from build123d import *

# Parameters (mm, degrees)
BOSS_EXTRUDE1_DEPTH = 7.9
SKETCH2_R           = 3.144549921
BOSS_EXTRUDE3_DEPTH = 0.5
SKETCH3_R           = 2.455888386
BOSS_EXTRUDE4_DEPTH = 7.9
SKETCH4_R           = 2.65462565
BOSS_EXTRUDE5_DEPTH = 0.3
SKETCH5_R           = 2.198604039
CUT_EXTRUDE1_DEPTH  = 7.9
CUT_EXTRUDE2_DEPTH  = 3.3
FILLET1_R           = 0.3
CUT_EXTRUDE5_START  = 9
SKETCH7_R           = 3.144549921
CUT_EXTRUDE5_DEPTH  = 9


with BuildPart() as part:
    # Sketch1 → Boss-Extrude1 (new body)
    with BuildSketch(Plane.XY):
        Polygon((-2.4, 0.895), (-2.4, 0), (0, 0), (0, 2.4), (-0.9, 2.4), (-0.9, 0.895), align=None)
        Polygon((0, 0), (-2.4, 0), (-2.4, -0.895), (-0.9, -0.895), (-0.9, -2.4), (0, -2.4), align=None)
        Polygon((0, 2.4), (0, 0), (2.4, 0), (2.4, 0.895), (0.9, 0.895), (0.9, 2.4), align=None)
        Polygon((2.4, 0), (0, 0), (0, -2.4), (0.9, -2.4), (0.9, -0.895), (2.4, -0.895), align=None)
    extrude(amount=BOSS_EXTRUDE1_DEPTH)

    # Sketch2 → Boss-Extrude3 (add)
    with BuildSketch(Plane(origin=(0, 0, 0), x_dir=(-1, 0, 0), z_dir=(0, 0, -1))):
        Circle(SKETCH2_R)
    extrude(amount=BOSS_EXTRUDE3_DEPTH)

    # Sketch3 → Boss-Extrude4 (add)
    with BuildSketch(Plane(origin=(0, 0, -0.5), x_dir=(-1, 0, 0), z_dir=(0, 0, -1))):
        Circle(SKETCH3_R)
    extrude(amount=BOSS_EXTRUDE4_DEPTH)

    # Sketch4 → Boss-Extrude5 (add)
    with BuildSketch(Plane(origin=(0, 0, -8.4), x_dir=(-1, 0, 0), z_dir=(0, 0, -1))):
        Circle(SKETCH4_R)
    extrude(amount=-BOSS_EXTRUDE5_DEPTH)

    # Sketch5 → Cut-Extrude1 (cut)
    with BuildSketch(Plane(origin=(0, 0, -8.4), x_dir=(-1, 0, 0), z_dir=(0, 0, -1))):
        Circle(SKETCH5_R)
    extrude(amount=-CUT_EXTRUDE1_DEPTH, mode=Mode.SUBTRACT)

    # Sketch6 → Cut-Extrude2 (cut)
    with BuildSketch(Plane(origin=(0, 0, -8.4), x_dir=(-1, 0, 0), z_dir=(0, 0, -1))):
        with BuildLine():
            Line((0.375484044, 2.166303638), (0.375484044, 2.627936276))
            ThreePointArc((0.375484044, 2.627936276), (0.188215694, 2.6479449), (0, 2.65462565))
            Line((0, 2.65462565), (0, 2.198604039))
            ThreePointArc((0, 2.198604039), (0.188435389, 2.190514055), (0.375484044, 2.166303638))
        make_face()
        with BuildLine():
            Line((0, 2.198604039), (0, 2.65462565))
            ThreePointArc((0, 2.65462565), (-0.188215694, 2.6479449), (-0.375484044, 2.627936276))
            Line((-0.375484044, 2.627936276), (-0.375484044, 2.166303638))
            ThreePointArc((-0.375484044, 2.166303638), (-0.188435389, 2.190514055), (0, 2.198604039))
        make_face()
        with BuildLine():
            ThreePointArc((0, -2.65462565), (0.188215694, -2.6479449), (0.375484044, -2.627936276))
            Line((0.375484044, -2.627936276), (0.375484044, -2.166303638))
            ThreePointArc((0.375484044, -2.166303638), (0, -2.198604039), (-0.375484044, -2.166303638))
            Line((-0.375484044, -2.166303638), (-0.375484044, -2.627936276))
            ThreePointArc((-0.375484044, -2.627936276), (-0.188215694, -2.6479449), (0, -2.65462565))
        make_face()
    extrude(amount=-CUT_EXTRUDE2_DEPTH, mode=Mode.SUBTRACT)

    # Fillet1
    fillet1_edges = [part.edges().sort_by_distance(p)[0] for p in [
        (0.375484044, 2.296659081, -5.1),
        (-0.375484044, 2.296659081, -5.1),
        (-0.375484044, -2.296659081, -5.1),
        (0.375484044, -2.296659081, -5.1),
    ]]
    fillet(fillet1_edges, radius=FILLET1_R)

    # Sketch7 → Cut-Extrude5 (cut)
    with BuildSketch(Plane.XY.offset(CUT_EXTRUDE5_START)):
        with Locations(Location((0, 0, 0), (0, 0, 180))):
            Circle(SKETCH7_R)
    extrude(amount=-CUT_EXTRUDE5_DEPTH, mode=Mode.SUBTRACT)

    # Mirror3: part across face


with BuildPart() as part_1:
    add(part.part)
    add(part.part.mirror(Plane.XY))


solid = part_1.part
Input: part model. Units: mm. Frame: model coordinates. A direction names the side the tool comes from. Coordinates: 2 decimals unless noted, no trailing zeros. Loops run counter-clockwise (first coordinate to the right, second up) from the corner with the lowest first, then second, coordinate; pieces in that order, holes last.
(1) Section B-B on y = 0. Return the cut outline in (x, z).
(2) Section A-A on z = 5.75. Return the cut outline in (x, y), then the cut area to 3 significant figures.
(3) Pull-direction query (Y, two-part tool) for faces 1 (the face through (2.4, 0.2, -8.4)), 2 (the face through (0.477, -2.146, 4.505)), 3 (the face through (0.68, -3.07, -0.01)); classes: released by +Y, released by -Y, zero draft, split by the parting line, or undercut.
(4) Section D-D on x = 2. Return the cut outline in (y, z), then the cut area to 3 significant figures.
(5) Set-up query: faces 4 (the face through (0, 0, 0.5)), 5 (the face through (2, -2, -0.5)), 6 (the face through (0.477, -2.146, -4.505)), 7 (the face through (-2.4, 0, 8.4)). Return all of +Z, -Z, +X, -X, +Y, -Y with unobstructed straight access to the full face (end or side cutting, diameter ignored); none if empty.
(6) Section C-C on z = -2. Return the cut outline in (x, y), then the cut area to 3 significant figures.
(7) Material intervals for probe 1 along Z at (x, y) = (-2.5, 0.25); probe 2 along Y at (x, z) = (0, 3.25); probe 3 along Z at (x, y) = (1.5, -1), sorted ascending.
(8) First-contact query: pin 1 Ø0.5 at (y, z) = (2.5, 7) entering from -X; pin 2 Ø2 at (y, z) = (-1.5, -2.5) entering from -X; pin 3 Ø0.7 at (x, y) = (-1, 0.5) entering from +Z. Flat tips, straight axial feed; report the tip coordinate or a pass-through.
Data:
1. outline: (-3.14, -0.5) - (-2.46, -0.5) - (-2.46, -8.1) - (-2.65, -8.1) - (-2.65, -8.4) - (-2.2, -8.4) - (-2.2, -0.5) - (2.2, -0.5) - (2.2, -8.4) - (2.65, -8.4) - (2.65, -8.1) - (2.46, -8.1) - (2.46, -0.5) - (3.14, -0.5) - (3.14, 0.5) - (2.46, 0.5) - (2.46, 8.1) - (2.65, 8.1) - (2.65, 8.4) - (2.2, 8.4) - (2.2, 0.5) - (-2.2, 0.5) - (-2.2, 8.4) - (-2.65, 8.4) - (-2.65, 8.1) - (-2.46, 8.1) - (-2.46, 0.5) - (-3.14, 0.5) - close
2. outline: (-0.38, -2.43) - (-0.38, -2.17) arc R2.2 cw to (-0.38, 2.17) - (-0.38, 2.43) arc R2.46 ccw to start; (0.38, -2.43) arc R2.46 ccw to (0.38, 2.43) - (0.38, 2.17) arc R2.2 cw to (0.38, -2.17) - close
2. area: 3.37 mm2
3. face 1: zero draft
3. face 2: undercut
3. face 3: split by the parting line
4. outline: (-2.43, -0.5) - (-1.43, -0.5) - (-1.43, -8.1) - (-1.75, -8.1) - (-1.75, -8.4) - (-0.91, -8.4) - (-0.91, -0.5) - (0.91, -0.5) - (0.91, -8.4) - (1.75, -8.4) - (1.75, -8.1) - (1.43, -8.1) - (1.43, -0.5) - (2.43, -0.5) - (2.43, 0.5) - (1.43, 0.5) - (1.43, 8.1) - (1.75, 8.1) - (1.75, 8.4) - (0.91, 8.4) - (0.91, 0.5) - (-0.91, 0.5) - (-0.91, 8.4) - (-1.75, 8.4) - (-1.75, 8.1) - (-1.43, 8.1) - (-1.43, 0.5) - (-2.43, 0.5) - close
4. area: 21.4 mm2
5. face 4: +Z
5. face 5: none
5. face 6: -Z
5. face 7: +Z, +X, -X, +Y, -Y
6. outline: circle Ø4.91 at (0, 0); hole circle Ø4.4 at (0, 0)
6. area: 3.76 mm2
7. probe 1: z = -8.4 to -8.1, -0.5 to 0.5, 8.1 to 8.4
7. probe 2: y = -2.46 to -2.2, 2.2 to 2.46
7. probe 3: z = -0.5 to 0.5
8. pin 1: stops at x = -0.98
8. pin 2: stops at x = -2.4
8. pin 3: stops at z = 0.5
